from build123d import *

# Parameters (mm, degrees)
SKETCH_2_R          = 9.5
SKETCH_2_R_2        = 1.25
SKETCH_2_R_3        = 13.25
SKETCH_2_R_4        = 2.1
EXTRUDE_1_DEPTH     = 3
SKETCH_4_R          = 1.6
CUT_EXTRUDE_1_DEPTH = 10
SKETCH_5_R          = 1.65
CUT_EXTRUDE_2_DEPTH = 10


with BuildPart() as part:
    # ｽｹｯﾁ2 → ﾎﾞｽ - 押し出し1 (new body)
    with BuildSketch(Plane.XY):
        with BuildLine():
            Line((-60, -22.5), (-40, -22.5))
            Line((-40, -22.5), (0, -22.5))
            ThreePointArc((0, -22.5), (15.909902577, -15.909902577), (22.5, 0))
            Line((22.5, 0), (22.5, 85))
            ThreePointArc((22.5, 85), (15.909902577, 100.909902577), (0, 107.5))
            Line((0, 107.5), (-40, 107.5))
            Line((-40, 107.5), (-60, 107.5))
            Line((-60, 107.5), (-60, -22.5))
        make_face()
        Circle(SKETCH_2_R, mode=Mode.SUBTRACT)
        with Locations((0, 17.5)):
            Circle(SKETCH_2_R_2, mode=Mode.SUBTRACT)
        with Locations((17.5, 0)):
            Circle(SKETCH_2_R_2, mode=Mode.SUBTRACT)
        with Locations((0, -17.5)):
            Circle(SKETCH_2_R_2, mode=Mode.SUBTRACT)
        with Locations((-17.5, 0)):
            Circle(SKETCH_2_R_2, mode=Mode.SUBTRACT)
        with Locations((0, 85)):
            Circle(SKETCH_2_R_3, mode=Mode.SUBTRACT)
        with Locations((0, 67.5)):
            Circle(SKETCH_2_R_4, mode=Mode.SUBTRACT)
        with Locations((-17.5, 85)):
            Circle(SKETCH_2_R_4, mode=Mode.SUBTRACT)
        with Locations((0, 102.5)):
            Circle(SKETCH_2_R_4, mode=Mode.SUBTRACT)
        with Locations((17.5, 85)):
            Circle(SKETCH_2_R_4, mode=Mode.SUBTRACT)
    extrude(amount=EXTRUDE_1_DEPTH)

    # ｽｹｯﾁ4 → ｶｯﾄ - 押し出し1 (cut)
    with BuildSketch(Plane.XY.offset(3)):
        with BuildLine():
            Line((-56.49, 77.55), (-60, 77.55))
            Line((-60, 77.55), (-60, 57.45))
            Line((-60, 57.45), (-56.49, 57.45))
            ThreePointArc((-56.49, 57.45), (-54.832182541, 57.332182541), (-54.95, 58.99))
            Line((-54.95, 58.99), (-54.95, 76.01))
            ThreePointArc((-54.95, 76.01), (-54.832182541, 77.667817459), (-56.49, 77.55))
        make_face()
        with BuildLine():
            Line((-56.49, 27.55), (-60, 27.55))
            Line((-60, 27.55), (-60, 7.45))
            Line((-60, 7.45), (-56.49, 7.45))
            ThreePointArc((-56.49, 7.45), (-54.832182541, 7.332182541), (-54.95, 8.99))
            Line((-54.95, 8.99), (-54.95, 26.01))
            ThreePointArc((-54.95, 26.01), (-54.832182541, 27.667817459), (-56.49, 27.55))
        make_face()
        with Locations((-57.5, 2.5)):
            Circle(SKETCH_4_R)
        with Locations((-57.5, 42.5)):
            Circle(SKETCH_4_R)
        with Locations((-57.5, 92.5)):
            Circle(SKETCH_4_R)
    extrude(amount=-CUT_EXTRUDE_1_DEPTH, mode=Mode.SUBTRACT)

    # ｽｹｯﾁ5 → ｶｯﾄ - 押し出し2 (cut)
    with BuildSketch(Plane.XY.offset(3)):
        with Locations((-9.5, 42.5)):
            Circle(SKETCH_5_R)
    extrude(amount=-CUT_EXTRUDE_2_DEPTH, mode=Mode.SUBTRACT)


solid = part.part
Source: CAD feature listing. Evaluate the final solid. Frame: model axes, mm. A direction names the side the tool comes from. Coordinates: 2 decimals unless noted, no trailing zeros. Order: outer loops, then holes, each group sorted by start corner. A loop starts at its lowest first (then second) coordinate and runs counter-clockwise, first axis right, second up.
Item 1: Cut plane C-C (z = 1.3). Count the separate pieces of the cut face and the enclosed holes in it, plus the area to 3 significant figures.
Output values:
separate pieces: 1
enclosed holes: 14
area: 9,360 mm2
Item 2: Cut plane A-A (y = 17.5). Return loops of the section in (x, z).
Output values:
outline: (-54.95, 0) - (-1.25, 0) - (-1.25, 3) - (-54.95, 3) - close; (1.25, 0) - (22.5, 0) - (22.5, 3) - (1.25, 3) - close
Item 3: Pull-direction query (Y, two-part tool) for faces 3 (the face through (-1.666, 66.222, 1.479)), 4 (the face through (16.084, 100.734, 1.479)), 5 (the face through (-30, -22.5, 1)), 6 (the face through (-19, 43, 0)); classes: pulls with the +Y half, pulls with the -Y half, needs draft (parallel to the pull), parting line crosses it, or undercut.
Output values:
face 3: undercut
face 4: pulls with the +Y half
face 5: pulls with the -Y half
face 6: needs draft
Item 4: Cut plane D-D (y = 92.5). Return loops of the section in (x, z).
Output values:
outline: (-60, 0) - (-59.1, 0) - (-59.1, 3) - (-60, 3) - close; (-55.9, 0) - (-10.92, 0) - (-10.92, 3) - (-55.9, 3) - close; (10.92, 0) - (21.21, 0) - (21.21, 3) - (10.92, 3) - close
Item 5: Set-up query: faces 1 (the face through (-58, 77.55, 2)), 2 (the face through (18.655, -0.479, 1.479)). Return all of +Z, -Z, +X, -X, +Y, -Y with unobstructed straight access to the full face (end or side cutting, diameter ignored); none if empty.
Output values:
face 1: +Z, -Z, -X
face 2: +Z, -Z
Item 6: First-contact query: P1, Ø1.9, axis at x = -57.5, y = 92.5, coming from the -Z side; P2, Ø0.9, axis at y = 71, z = 2, coming from the -X side. Flat tips, straight axial feed; report the tip coordinate or a pass-through.
Output values:
P1: passes through
P2: stops at x = -54.95
Item 7: Material intervals for line 1 (Y direction, x = -55.61, z = 2.3); line 2 (Y direction, x = 17.5, z = 0.95); line 3 (X direction, y = 76.89, z = 2), sorted ascending.
Output values:
line 1: y = -22.5 to 7.01, 27.99 to 57.01, 77.99 to 107.5
line 2: y = -14.14 to -1.25, 1.25 to 82.9, 87.1 to 99.14
line 3: x = -54.51 to -10.48, 10.48 to 22.5
Item 8: Cut plane B-B (x = -17.5). Return loops of the section in (y, z).
Output values:
outline: (-22.5, 0) - (-1.25, 0) - (-1.25, 3) - (-22.5, 3) - close; (1.25, 0) - (82.9, 0) - (82.9, 3) - (1.25, 3) - close; (87.1, 0) - (107.5, 0) - (107.5, 3) - (87.1, 3) - close
